```python
from build123d import *

# Parameters (mm, degrees)
CROQUIS2_W                 = 19.9
CROQUIS2_H                 = 19.9
SALIENTE_EXTRUIR1_DEPTH    = 5
CORTAR_EXTRUIR1_DEPTH      = 87.156862756
CORTAR_EXTRUIR1_DEPTH_BACK = 40
REDONDEO3_R                = 2
REDONDEO4_R                = 2


with BuildPart() as part:
    # Croquis1 → Revolución1 (revolve)
    with BuildSketch(Plane(origin=(0, 0, 0), x_dir=(0, 0, -1), z_dir=(1, 0, 0)), mode=Mode.PRIVATE) as revoluci_n1_sk:
        Polygon((0, 0), (-3.9, 0), (-3.9, 75), (-6, 75), (-6, 80), (0, 80), align=None)
    revolve(revoluci_n1_sk.sketch.rotate(Axis((0, 0, 0), (0, 1, 0)), 180), axis=Axis((0, 0, 0), (0, 1, 0)))

    # Croquis2 → Saliente-Extruir1 (add)
    with BuildSketch(Plane(origin=(0, 80, 0), x_dir=(1, 0, 0), z_dir=(0, 1, 0))):
        Rectangle(CROQUIS2_W, CROQUIS2_H)
    extrude(amount=SALIENTE_EXTRUIR1_DEPTH)

    # Croquis3 → Cortar-Extruir1 (cut, two sides: drawn at the far end of the back side and taken through both)
    with BuildSketch(Plane.XZ.offset(-CORTAR_EXTRUIR1_DEPTH_BACK)):
        Polygon((2, 49.105251298), (2, 3.348133809), (2, -3.348133809), (2, -49.105251298), (93.514234979, -49.105251298), (93.514234979, 49.105251298), align=None)
    extrude(amount=CORTAR_EXTRUIR1_DEPTH + CORTAR_EXTRUIR1_DEPTH_BACK, mode=Mode.SUBTRACT)

    # Redondeo3
    redondeo3_edges = [part.edges().sort_by_distance(p)[0] for p in [
        (0, 80, 6),
    ]]
    fillet(redondeo3_edges, radius=REDONDEO3_R)

    # Redondeo4
    redondeo4_edges = [part.edges().sort_by_distance(p)[0] for p in [
        (0, 80, 9.95),
        (9.95, 80, 0),
        (-9.95, 80, 0),
        (0, 80, -9.95),
    ]]
    fillet(redondeo4_edges, radius=REDONDEO4_R)


solid = part.part
```
Here's how the part is built. I have some questions about the finished solid (model axes, mm). A direction names the side the tool comes from. Round coordinates to 2 decimals unless told otherwise and drop trailing zeros. Loops run counter-clockwise (first coordinate to the right, second up) from the corner with the lowest first, then second, coordinate; pieces in that order, holes last. Notation, with made-up numbers: (-7, 6.5) -> (46, 6.5) arc R19 ccw to (46, 20.5) -> close; hole circle Ø8 at (47.25, 31.5). An arc over 180 degrees is marked (long way). Answer as CSV lines item,"result". Start each with the question number.
1. I'm going to push flat-ended pins straight in: P1, Ø3.5, axis at x = -6, z = -6, coming from the -Y side; P2, Ø1.5, axis at y = 46.5, z = -0.5, coming from the +X side; P3, Ø5, axis at y = 13, z = 5.5, coming from the -X side. Where does each tip first touch, or does it pass through?
2. Imagine slicing it at A-A on y = 58. Write out the boundary of the cut face in (x, z).
3. For faces 1 (the face through (-3.288, 38.025, -2.097)), 2 (the face through (6, 80, -6)), 3 (the face through (3, 40, 0)), 4 (the face through (-6, 80, 6)), 5 (the face through (6, 80, 6)), which set-ups out of +Z, -Z, +X, -X, +Y, -Y let a thin tool reach every point of the face, with its end or its side?
4. I need wall thicknesses on probe 1 along Z at (x, y) = (-2, 9); probe 2 along Y at (x, z) = (2.75, 8); probe 3 along Y at (x, z) = (3, 1.5). Which ranges of each line are inside material? Lowest first, please. Write a range as from..to.
Solution:
1,P1,"y = 79.55"
1,P2,"x = 3.9"
1,P3,"x = -2.49"
2,outline,"circle Ø7.8 at (0, 0)"
3,face 1,"-Y"
3,face 2,"-Z, +X, -Y"
3,face 3,"+Z, -Z, +X, -Y"
3,face 4,"+Z, -X, -Y"
3,face 5,"+Z, +X, -Y"
4,probe 1,"-3.35..3.35"
4,probe 2,"80..85"
4,probe 3,"40..85"
